Verification items for the finished model (mm, model axes). Face numbers are marked on the shaded views. A direction names the side the tool comes from. Coordinates: 2 decimals unless noted, no trailing zeros. Write each loop counter-clockwise with the first axis right and the second up, starting at its lowest first coordinate (ties: lowest second). Pieces come first, ordered by that corner, then holes. Notation, with made-up numbers: (32, 59) -> (43, 59) arc R22 cw to (43, 83) -> close; hole circle Ø7 at (-36.75, 46). An arc over 180 degrees is marked (long way). Answer in a Markdown table with one row per item.
Autodesk Inventor part; units mm, degrees
ref_plane "YZ Plane" through (0, 0, 0) normal (1, 0, 0) x (0, 1, 0)
ref_plane "XZ Plane" through (0, 0, 0) normal (0, 1, 0) x (-1, 0, 0)
ref_plane "XY Plane" through (0, 0, 0) normal (0, 0, 1) x (1, 0, 0)
sketch "Sketch1" plane through (0, 0, 0) normal (0, 0, 1) x (1, 0, 0)
  line L0 (21, -21) -> (-21, -21)
  line L1 (-21, -21) -> (-21, 21)
  line L2 (-21, 21) -> (21, 21)
  line L3 (21, 21) -> (21, -21)
  line L4 (21, -21) -> (-21, 21) construction
  line L5 (-21, -21) -> (21, 21) construction
  point P0 (0, 0)
  dimension "d0" = 42
extrude "Extrusion1" add sketch "Sketch1" along normal blind 30
sketch "Sketch2" plane through (0, 0, 30) normal (0, 0, 1) x (1, 0, 0)
  point P0 (0, 0)
  point P1 (-15.5, 15.5)
  point P2 (-15.5, -15.5)
  point P3 (15.5, -15.5)
  point P4 (15.5, 15.5)
  dimension "d3" = 31
  dimension "d4" = 31
  dimension "d5" = 15.5
  dimension "d6" = 15.5
hole "Hole1" at (-15.5, 15.5, 30) at (-15.5, -15.5, 30) at (15.5, -15.5, 30) at (15.5, 15.5, 30) direction (0, 0, -1) diameter 3 depth 8 tip angle 118
chamfer "Chamfer1" distance 3.5 angle 45 4 edges at (21, 21, 15) (21, -21, 15) (-21, 21, 15) (-21, -21, 15)
sketch "Sketch3" plane through (0, 0, 30) normal (0, 0, 1) x (1, 0, 0)
  circle A0 centre (0, 0) radius 11
  dimension "d17" = 22
extrude "Extrusion2" add sketch "Sketch3" along normal blind 2
sketch "Sketch4" plane through (0, 0, 32) normal (0, 0, 1) x (1, 0, 0)
  circle A0 centre (0, 0) radius 11
  circle A1 centre (0, 0) radius 2.5
  dimension "d20" = 5
extrude "Extrusion3" add sketch "Sketch4" along normal blind 25 contours A1
properties part number "Extruder Motor" material "Steel, Alloy"
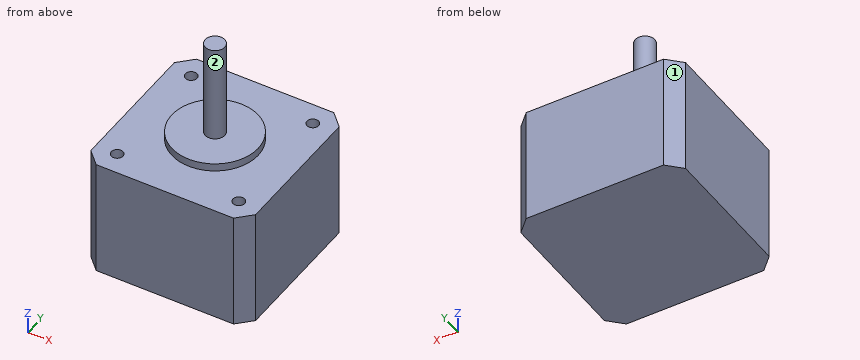
1. Sectioned sample at A-A, the plane y = 0. Record the cut outline in (x, z), and give its area (3 significant figures).
Findings below:
| item | result |
|---|---|
| outline | (-21, 0) -> (21, 0) -> (21, 30) -> (11, 30) -> (11, 32) -> (2.5, 32) -> (2.5, 57) -> (-2.5, 57) -> (-2.5, 32) -> (-11, 32) -> (-11, 30) -> (-21, 30) -> close |
| area | 1,430 mm² |
2. Material ranges on probe 1 along X at (y, z) = (15.5, 25); probe 2 along X at (y, z) = (-15, 26), recorded low to high. Write a range as from..to.
Findings below:
| item | result |
|---|---|
| probe 1 | x = -21..-17, -14..14, 17..21 |
| probe 2 | x = -21..-16.91, -14.09..14.09, 16.91..21 |
3. Sectioned sample at D-D, the plane y = -13. Record the cut outline in (x, z).
Findings below:
| item | result |
|---|---|
| outline | (-21, 0) -> (21, 0) -> (21, 30) -> (-21, 30) -> close |
4. Sectioned sample at B-B, the plane x = -5. Record the cut outline in (y, z).
Findings below:
| item | result |
|---|---|
| outline | (-21, 0) -> (21, 0) -> (21, 30) -> (9.8, 30) -> (9.8, 32) -> (-9.8, 32) -> (-9.8, 30) -> (-21, 30) -> close |
5. Sectioned sample at C-C, the plane z = 45. Record the cut outline in (x, y), and give its area (3 significant figures).
Findings below:
| item | result |
|---|---|
| outline | circle Ø5 at (0, 0) |
| area | 19.6 mm² |
6. Go/stop test with flat-tipped pins: pin 1 (2.5 mm diameter, centred on x = -15.5, y = 15.5, fed in from +Z); pin 2 (1 mm diameter, centred on x = -16, y = 0, fed in from +Z); pin 3 (10 mm diameter, centred on x = 5, y = -12.5, fed in from +Z). Record where each tip stops, or that it passes through.
Findings below:
| item | result |
|---|---|
| pin 1 | stops at z = 21.85 |
| pin 2 | stops at z = 30 |
| pin 3 | stops at z = 32 |
7. Access from +Z, -Z, +X, -X, +Y, -Y to the whole of each face (thin tool, end or side, straight path). Record for the marked faces 1 and 2.
Findings below:
| item | result |
|---|---|
| face 1 | +Z, -Z, -X, +Y |
| face 2 | +Z |
